The listing builds one solid part. Answer for the finished solid, in the listing's coordinates (mm). A direction names the side the tool comes from. Give positions to 0.01 mm unless a question says otherwise; leave off trailing zeros. Loops run counter-clockwise (first coordinate to the right, second up) from the corner with the lowest first, then second, coordinate; pieces in that order, holes last. Notation, with made-up numbers: M 44.5,9.5 L 100.5,9.5 A14 ccw 100.5,24.5 Z; hole C -12,44 d9. An arc over 180 degrees is marked long. One line per item, written item: value. Start each with the question number.
Q1. The mould has two halves that part along X. Classify faces 1 (the cylindrical face through (14.248, -76.287, 55.064)), 2 (the flat face through (-22, -73, 55)), 3 (the cylindrical face through (23.82, -75.96, 56.08)), 4 (the flat face through (-29.5, -76, 55)): +X half, -X half, draft (parallel to the pull), parting line (faces both ways), or undercut.
Q2. A cutting plane is placed at C-C, the plane x = 3.5. Determine the outline of the cut face in (y, z).
Q3. A cutting plane is placed at B-B, the plane z = 55. State how many separate pieces and enclosed holes the cut face has, and give its area (3 significant figures).
Q4. For faces 5 (the flat face through (0, -78, 60)), 6 (the flat face through (0, -77, 55)), 7 (the conical face through (14.324, -76.365, 50.292)), determine the directions among +Z, -Z, +X, -X, +Y, -Y from which every point of the face is accessible in a straight line to the end or side of a thin tool.
Q5. A cutting plane is placed at D-D, the plane z = 51.25. Determine the outline of the cut face in (x, y).
Q6. A cutting plane is placed at A-A, the plane x = -25. Determine the outline of the cut face in (y, z).
Q7. Consider L1, parallel to X at y = -76, z = 56; L2, parallel to X at y = -77.75, z = 54.25; L3, parallel to X at y = -74, z = 59. Determine where each line is inside the solid, lowest interval first.
Q8. A flat-ended cylindrical pin translates along its axis: pin 1 (3 mm diameter, centred on x = 11, z = 56, fed in from +Y). Find the tip coordinate at first contact, or state that the pin passes through.
from build123d import *

# Parameters (mm, degrees)
SKETCH134_W     = 59
SKETCH134_H     = 10
SKETCH134_R     = 1.6
PAD068_DEPTH    = 6
SKETCH135_W     = 30
SKETCH135_H     = 4
POCKET066_DEPTH = 7.5
FILLET048_R     = 2.5
CHAMFER053_SIZE = 0.6
CHAMFER054_SIZE = 0.4
CHAMFER055_SIZE = 0.4


with BuildPart() as part:
    # Sketch134 → Pad068 (new body)
    with BuildSketch(Plane.XZ):
        Rectangle(SKETCH134_W, SKETCH134_H)
        with Locations((-25, 0)):
            Circle(SKETCH134_R, mode=Mode.SUBTRACT)
        with Locations((25, 0)):
            Circle(SKETCH134_R, mode=Mode.SUBTRACT)
    extrude(amount=PAD068_DEPTH)

    # Sketch135 → Pocket066 (cut, symmetric)
    with BuildSketch(Plane.XY):
        with Locations((0, -2)):
            Rectangle(SKETCH135_W, SKETCH135_H)
    extrude(amount=POCKET066_DEPTH, both=True, mode=Mode.SUBTRACT)

    # Fillet048
    fillet048_edges = [part.edges().sort_by_distance(p)[0] for p in [
        (15, -4, 0),
        (-15, -4, 0),
    ]]
    fillet(fillet048_edges, radius=FILLET048_R)

    # Chamfer053
    chamfer053_edges = [part.edges().sort_by_distance(p)[0] for p in [
        (15, 0, 0),
        (-15, 0, 0),
        (29.5, 0, 0),
        (29.5, -6, 0),
        (-29.5, -6, 0),
        (-29.5, 0, 0),
    ]]
    chamfer(chamfer053_edges, length=CHAMFER053_SIZE)

    # Chamfer054
    chamfer054_edges = [part.edges().sort_by_distance(p)[0] for p in [
        (26.6, -3, 0),
        (23.4, 0, 0),
        (23.4, -6, 0),
        (-23.4, -3, 0),
        (-26.6, 0, 0),
        (-26.6, -6, 0),
    ]]
    chamfer(chamfer054_edges, length=CHAMFER054_SIZE)

    # Chamfer055
    chamfer055_edges = [part.edges().sort_by_distance(p)[0] for p in [
        (-15, -1.05, 5),
        (-15.3, -0.3, 5),
        (-14.267767, -3.267767, 5),
        (-22.25, 0, 5),
        (0, -4, 5),
        (-29.2, -0.3, 5),
        (14.267767, -3.267767, 5),
        (-29.5, -3, 5),
        (15, -1.05, 5),
        (-29.2, -5.7, 5),
        (15.3, -0.3, 5),
        (0, -6, 5),
        (22.25, 0, 5),
        (29.2, -5.7, 5),
        (29.2, -0.3, 5),
        (29.5, -3, 5),
        (15, -1.05, -5),
        (15.3, -0.3, -5),
        (14.267767, -3.267767, -5),
        (22.25, 0, -5),
        (0, -4, -5),
        (29.2, -0.3, -5),
        (-14.267767, -3.267767, -5),
        (29.5, -3, -5),
        (-15, -1.05, -5),
        (29.2, -5.7, -5),
        (-15.3, -0.3, -5),
        (0, -6, -5),
        (-22.25, 0, -5),
        (-29.2, -5.7, -5),
        (-29.2, -0.3, -5),
        (-29.5, -3, -5),
    ]]
    chamfer(chamfer055_edges, length=CHAMFER055_SIZE)


with BuildPart() as part_1:
    # Body051 placement: moved
    add(part.part.moved(Location((0, -73, 55))))


solid = part_1.part
Answer block:
1. face 1: undercut
1. face 2: draft
1. face 3: undercut
1. face 4: -X half
2. outline: M -79,50.4 L -78.6,50 L -77.4,50 L -77,50.4 L -77,59.6 L -77.4,60 L -78.6,60 L -79,59.6 Z
3. separate pieces: 3
3. enclosed holes: 0
3. area: 197 mm^2
4. face 5: +Z, +X, -X, +Y, -Y
4. face 6: +Z, -Z, +Y
4. face 7: -Z, +Y
5. outline: M -29.5,-78.4 L -28.9,-79 L 28.9,-79 L 29.5,-78.4 L 29.5,-73.6 L 28.9,-73 L 15.6,-73 L 15,-73.6 L 15,-74.5 A2.5 cw 12.5,-77 L -12.5,-77 A2.5 cw -15,-74.5 L -15,-73.6 L -15.6,-73 L -28.9,-73 L -29.5,-73.6 Z
6. outline: M -79,50.4 L -78.6,50 L -73.4,50 L -73,50.4 L -73,53 L -73.4,53.4 L -78.6,53.4 L -79,53 Z; M -79,57 L -78.6,56.6 L -73.4,56.6 L -73,57 L -73,59.6 L -73.4,60 L -78.6,60 L -79,59.6 Z
7. L1: -29.5 to -26.25, -23.75 to -14.5, 14.5 to 23.75, 26.25 to 29.5
7. L2: -29.5 to -26.41, -23.59 to 23.59, 26.41 to 29.5
7. L3: -29.5 to -15, 15 to 29.5
8. pin 1: y = -77
